Build history of the part. All positions in model axes, mm. A direction names the side the tool comes from. Give positions to 0.01 mm unless a question says otherwise; leave off trailing zeros. Loops run counter-clockwise (first coordinate to the right, second up) from the corner with the lowest first, then second, coordinate; pieces in that order, holes last. Notation, with made-up numbers: M -4.5,45.5 L 31.5,45.5 A12 ccw 31.5,67.5 Z; hole C 51.25,-22.5 d2. An arc over 180 degrees is marked long. Answer as a JSON object with one key per item and string values. Group by question number.
1. Mould opens along Z. For faces 1 (the face through (7, -6, 4)), 2 (the face through (-10.33, 10.31, 2.86)), 3 (the face through (3.3, -3.3, 3.5)) say: released by +Z, released by -Z, zero draft, split by the parting line, or undercut.
2. Slice it at B-B (x = 2). List the corners of the cut face in (y, z).
3. Drill centre lines: line 1 along Y through (x, z) = (-7.65, 0.2); line 2 along Z through (x, y) = (-4.5, 0); line 3 along Z through (x, y) = (-0.5, -0.75). Where is each one in solid material? Low to high. Write a range as [from, to].
4. Slice it at D-D (x = -3.5). List the corners of the cut face in (y, z), then the cut area to 3 significant figures.
5. 3-axis set-ups, long thin cutter, end or side, ignore diameter. For faces 4 (the face through (6, -7, 4)), 5 (the face through (-7, -6, 4)), 6 (the face through (10.36, -10.38, 2.25)): which of +Z, -Z, +X, -X, +Y, -Y reach the whole face in a straight line?
6. Slice it at A-A (y = 0). List the corners of the cut face in (x, z).
7. Drop flat-ended pins along their axis: pin 1 Ø1.6 at (y, z) = (1.5, 6.5) entering from -X; pin 2 Ø0.6 at (x, z) = (1.5, 6.5) entering from -Y; pin 3 Ø0.6 at (y, z) = (0.5, 5.5) entering from +X. Give the stop position or say it passes through.
8. Slice it at C-C (z = 4.25). List the corners of the cut face in (x, y), then the cut area to 3 significant figures.
from build123d import *

# Parameters (mm, degrees)
SKETCH_W           = 23
SKETCH_H           = 23
SKETCH_R           = 1.75
PAD_DEPTH          = 2
FILLET_R           = 1
CHAMFER_SIZE       = 1
PAD002_DEPTH       = 3.8
CHAMFER002_SIZE    = 1
SKETCH003_W        = 1.414214
SKETCH003_H        = 6.9
PAD003_DEPTH       = 10
POLARPATTERN_COUNT = 4
CHAMFER003_SIZE    = 4
SKETCH004_W        = 2.365725
SKETCH004_H        = 2.9
POCKET_DEPTH       = 11.501
POCKET_DEPTH_BACK  = -11.501
FILLET001_R        = 1


with BuildPart() as part:
    # Sketch → Pad (new body)
    with BuildSketch(Plane.XY):
        Rectangle(SKETCH_W, SKETCH_H)
        with Locations((-7.65, 0)):
            Circle(SKETCH_R, mode=Mode.SUBTRACT)
        with Locations((7.65, 0)):
            Circle(SKETCH_R, mode=Mode.SUBTRACT)
    extrude(amount=PAD_DEPTH)

    # Fillet
    fillet_edges = [part.edges().sort_by_distance(p)[0] for p in [
        (-11.5, 11.5, 1),
        (-11.5, -11.5, 1),
        (11.5, -11.5, 1),
        (11.5, 11.5, 1),
    ]]
    fillet(fillet_edges, radius=FILLET_R)

    # Chamfer
    chamfer_edges = [part.edges().sort_by_distance(p)[0] for p in [
        (-9.4, 0, 2),
        (5.9, 0, 2),
    ]]
    chamfer(chamfer_edges, length=CHAMFER_SIZE)

    # Sketch002 → Pad002 (join, symmetric)
    with BuildSketch(Plane.XZ):
        Polygon((-3.8, 6.9), (3.8, 6.9), (3.8, 4.9), (0.340708, 4.9), (0.340708, 0), (-0.340708, 0), (-0.340708, 4.9), (-3.8, 4.9), align=None)
    extrude(amount=PAD002_DEPTH, both=True)

    # Chamfer002
    chamfer002_edges = [part.edges().sort_by_distance(p)[0] for p in [
        (-3.8, -3.8, 5.9),
        (-3.8, 3.8, 5.9),
        (3.8, -3.8, 5.9),
        (3.8, 3.8, 5.9),
    ]]
    chamfer(chamfer002_edges, length=CHAMFER002_SIZE)

    # Sketch003 (on Face3 of Chamfer002) → Pad003 (join)
    with BuildSketch(Plane(origin=(-3.3, -3.3, 0), x_dir=(0.707107, -0.707107, 0), z_dir=(-0.707107, -0.707107, 0))):
        with Locations((0, 3.45)):
            Rectangle(SKETCH003_W, SKETCH003_H)
    pad003 = extrude(amount=PAD003_DEPTH)

    # PolarPattern: Pad003 ×4 about axis
    polarpattern_axis = Axis((0, 0, 0), (0, 0, 1))
    for i in range(1, POLARPATTERN_COUNT):
        add(pad003.rotate(polarpattern_axis, i * 360 / POLARPATTERN_COUNT))

    # Chamfer003
    chamfer003_edges = [part.edges().sort_by_distance(p)[0] for p in [
        (10.371068, -10.371068, 6.9),
        (10.371068, 10.371068, 6.9),
        (-10.371068, 10.371068, 6.9),
        (-10.371068, -10.371068, 6.9),
    ]]
    chamfer(chamfer003_edges, length=CHAMFER003_SIZE)

    # Sketch004 → Pocket (cut, two sides)
    with BuildSketch(Plane.XZ) as pocket_sk:
        with Locations((0.122459, 3.45)):
            Rectangle(SKETCH004_W, SKETCH004_H)
    extrude(amount=-POCKET_DEPTH, mode=Mode.SUBTRACT)
    extrude(pocket_sk.sketch, amount=-POCKET_DEPTH_BACK, mode=Mode.SUBTRACT)

    # Fillet001
    fillet001_edges = [part.edges().sort_by_distance(p)[0] for p in [
        (-10.371068, -10.371068, 2.9),
        (10.371068, -10.371068, 2.9),
        (7.542641, -7.542641, 6.9),
        (-7.542641, -7.542641, 6.9),
        (-7.542641, 7.542641, 6.9),
        (7.542641, 7.542641, 6.9),
        (10.371068, 10.371068, 2.9),
        (-10.371068, 10.371068, 2.9),
    ]]
    fillet(fillet001_edges, radius=FILLET001_R)


solid = part.part
Established:
{
 "1": {"face 1": "zero draft", "face 2": "released by +Z", "face 3": "undercut"},
 "2": {"outline": "M -11.5,0 L 11.5,0 L 11.5,2 L -11.5,2 Z; M -3.8,4.9 L 3.8,4.9 L 3.8,6.9 L -3.8,6.9 Z"},
 "3": {"line 1": "y = [-11.5, -1.75], [1.75, 11.5]", "line 2": "z = [0, 2]", "line 3": "z = [0, 2], [4.9, 6.9]"},
 "4": {"outline": "M -11.5,0 L 11.5,0 L 11.5,2 L 4.5,2 L 4.5,6.9 L -4.5,6.9 L -4.5,2 L -11.5,2 Z; hole M -3.1,2 L 3.1,2 L 3.1,4.9 L -3.1,4.9 Z", "area": "72.1 mm^2"},
 "5": {"face 4": "+Z, -Y", "face 5": "+Z, -X", "face 6": "+Z, +X, -Y"},
 "6": {"outline": "M -11.5,0 L -9.4,0 L -9.4,1 L -10.4,2 L -11.5,2 Z; M -5.9,0 L 5.9,0 L 5.9,1 L 4.9,2 L -4.9,2 L -5.9,1 Z; M -3.8,4.9 L 3.8,4.9 L 3.8,6.9 L -3.8,6.9 Z; M 9.4,0 L 11.5,0 L 11.5,2 L 10.4,2 L 9.4,1 Z"},
 "7": {"pin 1": "stops at x = -3.8", "pin 2": "stops at y = -3.8", "pin 3": "stops at x = 3.8"},
 "8": {"outline": "M -9.92,-8.92 L -8.92,-9.92 L -2.8,-3.8 L -3.8,-2.8 Z; M -9.92,8.92 L -3.8,2.8 L -2.8,3.8 L -8.92,9.92 Z; M 2.8,-3.8 L 8.92,-9.92 L 9.92,-8.92 L 3.8,-2.8 Z; M 2.8,3.8 L 3.8,2.8 L 9.92,8.92 L 8.92,9.92 Z", "area": "48.9 mm^2"}
}
